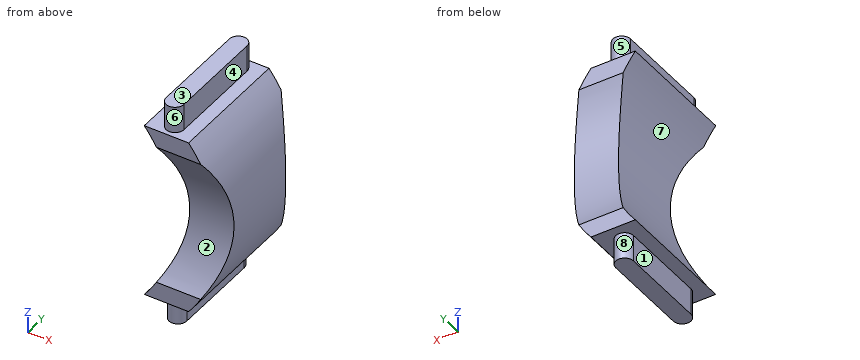
```python
from build123d import *

# Parameters (mm, degrees)
F1_DEPTH = 88.9
F3_DEPTH = 19.05
F5_DEPTH = 19.05
F8_DEPTH = 54.0395254203


with BuildPart() as f1:
    # F0 (on Front) → F1 (new body)
    with BuildSketch(Plane.XZ):
        with BuildLine():
            Line((-32.5461814261, -20.7940909142), (-32.5461814261, 106.2059090858))
            Line((-32.5461814261, 106.2059090858), (-64.2961814261, 106.2059090858))
            ThreePointArc((-64.2961814261, 106.2059090858), (-42.0076560058, 42.7059090858), (-64.2961814261, -20.7940909142))
            Line((-64.2961814261, -20.7940909142), (-32.5461814261, -20.7940909142))
        make_face()
        with BuildLine():
            ThreePointArc((-32.5461814261, -20.7940909142), (-10.2576560058, 42.7059090858), (-32.5461814261, 106.2059090858))
            Line((-32.5461814261, 106.2059090858), (-32.5461814261, -20.7940909142))
        make_face()
    extrude(amount=F1_DEPTH)

    # F2 (on face) → F3 (join)
    with BuildSketch(Plane(origin=(0, 0, -20.7940909142), x_dir=(1, 0, 0), z_dir=(0, 0, -1))):
        with BuildLine():
            Line((-42.0711814261, 12.7), (-42.0711814261, 76.2))
            ThreePointArc((-42.0711814261, 76.2), (-48.4211814261, 82.55), (-54.7711814261, 76.2))
            Line((-54.7711814261, 76.2), (-54.7711814261, 12.7))
            ThreePointArc((-54.7711814261, 12.7), (-48.4211814261, 6.35), (-42.0711814261, 12.7))
        make_face()
    extrude(amount=F3_DEPTH)

    # F4 (on face) → F5 (join)
    with BuildSketch(Plane.XY.offset(106.2059090858)):
        with BuildLine():
            Line((-42.0711817384, -79.375), (-42.0711817384, -9.525))
            ThreePointArc((-42.0711817384, -9.525), (-48.4211817384, -3.175), (-54.7711817384, -9.525))
            Line((-54.7711817384, -9.525), (-54.7711817384, -79.375))
            ThreePointArc((-54.7711817384, -79.375), (-48.4211817384, -85.725), (-42.0711817384, -79.375))
        make_face()
    extrude(amount=F5_DEPTH)

    # F7 (on 3pt) → F8 (cut, through all)
    with BuildSketch(Plane(origin=(-64.2961814261, 0, 0), x_dir=(0, -1, 0), z_dir=(-1, 0, 0))):
        with BuildLine():
            Line((-11.4886816591, -8.6150756106), (0, -8.0940909142))
            ThreePointArc((0, -8.0940909142), (15.875, 42.7059090858), (0, 93.5059090858))
            Line((0, 93.5059090858), (-11.4886816591, 93.5059090858))
            Line((-11.4886816591, 93.5059090858), (-11.4886816591, -8.6150756106))
        make_face()
        with BuildLine():
            ThreePointArc((88.9, 93.5059090858), (73.025, 42.7059090858), (88.9, -8.0940909142))
            Line((88.9, -8.0940909142), (100.3886816591, -8.6150756106))
            Line((100.3886816591, -8.6150756106), (100.3886816591, 93.5059090858))
            Line((100.3886816591, 93.5059090858), (88.9, 93.5059090858))
        make_face()
    extrude(amount=-F8_DEPTH, mode=Mode.SUBTRACT)


solid = f1.part
```
Source: CAD feature listing. Evaluate the final solid. Frame: model axes, mm. Face numbers are marked on the shaded views. A direction names the side the tool comes from. Coordinates: 2 decimals unless noted, no trailing zeros. Loops run counter-clockwise (first coordinate to the right, second up) from the corner with the lowest first, then second, coordinate; pieces in that order, holes last. Notation, with made-up numbers: M 7.5,36.25 L 38.5,36.25 A11 ccw 38.5,42.25 Z; hole C 23.5,60 d7. An arc over 180 degrees is marked long. Use a Markdown table: item, result. Add a question column.
Q1. Draft query along Z for the marked faces 1, 2 and 3. Return one class per face: pulls with the +Z half, pulls with the -Z half, needs draft (parallel to the pull), parting line crosses it, or undercut.
Q2. Section query C-C, the plane x = -50.5. Return loops of the section in (y, z) (1 decimal), and give its area (3 significant figures).
Q3. Access query for the marked faces 4, 5, 6, 7 and 8. Directions: +Z, -Z, +X, -X, +Y, -Y. A direction counts if a zero-diameter tool reaches every point of the face in a straight line with its end or side. Return the directions, or none.
Q4. Material intervals for L1, parallel to Z at x = -36.5, y = -44.5; L2, parallel to Y at x = -18, z = 45; L3, parallel to Z at x = -57, y = -34.5, sorted ascending.
Q5. Section query A-A, the plane y = -30.5. Return loops of the section in (x, z), and give its area (3 significant figures).
Q6. First-contact query: pin 1 (21 mm diameter, centred on y = -43.5, z = 117, fed in from -X); pin 2 (8 mm diameter, centred on y = -20, z = 33, fed in from +X); pin 3 (1 mm diameter, centred on y = -39, z = 75.5, fed in from +X). Flat tips, straight axial feed; report the tip coordinate or a pass-through.
Q7. Section query B-B, the plane x = -37.5. Return loops of the section in (y, z) (1 decimal).
Q8. Section query D-D, the plane z = 22.5. Return loops of the section in (x, y).
Result:
| question | item | result |
|---|---|---|
| 1 | face 1 | needs draft |
| 1 | face 2 | undercut |
| 1 | face 3 | pulls with the +Z half |
| 2 | outline | M -88.9,-20.8 L -82.2,-20.8 L -82.2,-39.8 L -6.7,-39.8 L -6.7,-20.8 L 0,-20.8 L 0,-8.1 A89.2 cw -6.1,2 L -82.8,2 A89.2 cw -88.9,-8.1 Z; M -88.9,93.5 A89.2 cw -82.8,83.4 L -6.1,83.4 A89.2 cw 0,93.5 L 0,106.2 L -3.5,106.2 L -3.5,125.3 L -85.4,125.3 L -85.4,106.2 L -88.9,106.2 Z |
| 2 | area | 6,930 mm2 |
| 3 | face 4 | +Z, +X, +Y, -Y |
| 3 | face 5 | +Z, +Y |
| 3 | face 6 | +Z, -Y |
| 3 | face 7 | -X, +Y, -Y |
| 3 | face 8 | -Z, +Y |
| 4 | L1 | z = -20.79 to 106.21 |
| 4 | L2 | y = -73.05 to -15.85 |
| 4 | L3 | z = -20.79 to -10.41, 95.83 to 106.21 |
| 5 | outline | M -64.3,-20.79 L -54.77,-20.79 L -54.77,-39.84 L -42.07,-39.84 L -42.07,-20.79 L -32.55,-20.79 A101.6 ccw -32.55,106.21 L -42.07,106.21 L -42.07,125.26 L -54.77,125.26 L -54.77,106.21 L -64.3,106.21 A101.6 cw Z |
| 5 | area | 4,520 mm2 |
| 6 | pin 1 | stops at x = -54.77 |
| 6 | pin 2 | stops at x = -10.42 |
| 6 | pin 3 | stops at x = -15.53 |
| 7 | outline | M -88.9,-20.8 L 0,-20.8 L 0,-8.1 A89.2 cw 0,93.5 L 0,106.2 L -88.9,106.2 L -88.9,93.5 A89.2 cw -88.9,-8.1 Z |
| 8 | outline | M -44.04,-75.34 L -12.29,-75.34 L -12.29,-13.56 L -44.04,-13.56 Z |
